from build123d import *

# Parameters (mm, degrees)
F0_W     = 69.85
F0_H     = 120.65
F0_W_2   = 9.525
F0_H_2   = 25.4
F1_DEPTH = 6.35
F3_R     = 11.90625
F4_DEPTH = 12.7
F2_R     = 11.90625
F5_DEPTH = 12.7
F6_W     = 11.43
F6_H     = 88.9
F7_DEPTH = 12.7


with BuildPart() as f1:
    # F0 (on Front) → F1 (new body)
    with BuildSketch(Plane.XZ):
        Rectangle(F0_W, F0_H)
        Rectangle(F0_W_2, F0_H_2, mode=Mode.SUBTRACT)
    extrude(amount=F1_DEPTH)

    # F3 (on Front) → F4 (join)
    with BuildSketch(Plane.XZ):
        with Locations((18.782835, 26.751311)):
            Circle(F3_R)
    extrude(amount=F4_DEPTH)

    # F2 (on Front) → F5 (join)
    with BuildSketch(Plane.XZ):
        with Locations((-17.48186, -7.399299)):
            Circle(F2_R)
    extrude(amount=F5_DEPTH)

    # F6 (on Front) → F7 (join)
    with BuildSketch(Plane.XZ):
        Rectangle(F6_W, F6_H)
    extrude(amount=F7_DEPTH)


solid = f1.part
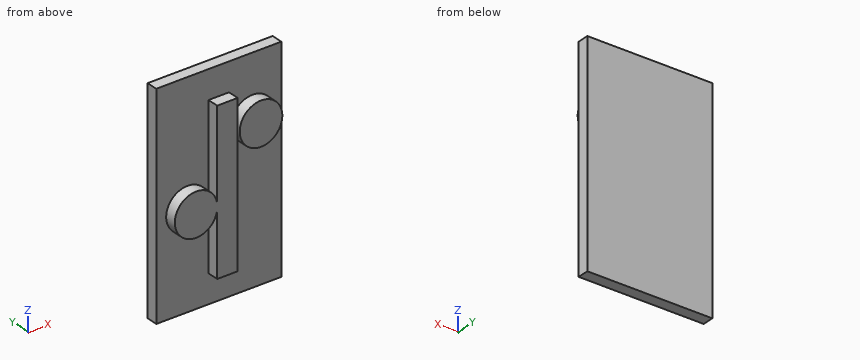
Work out the finished part from the listing and answer in its coordinate system (mm). Coordinates: 2 decimals unless noted, no trailing zeros. Loops run counter-clockwise (first coordinate to the right, second up) from the corner with the lowest first, then second, coordinate; pieces in that order, holes last. Notation, with made-up numbers: M 36.5,63 L 40.5,63 A13 cw 40.5,68 Z; hole C 32,34.25 d7. An arc over 180 degrees is marked long. Answer in a Markdown table with one row per item. Add a question column.
1. Flat-ended cylindrical pins translate along their axes: P1, Ø1, axis at x = 17, y = -8.5, coming from the -Z side; P2, Ø3, axis at x = 1, y = -8.5, coming from the +Z side; P3, Ø5, axis at y = -11, z = -19.5, coming from the -X side; P4, Ø7, axis at y = -9, z = 26.5, coming from the -X side (3 decimals). Find the tip coordinate at first contact, or state that the pin passes through.
2. Find section D-D, the plane z = 36. Write down the section's boundary in (x, y) (3 decimals), then the cut area to 3 significant figures.
3. Find section A-A, the plane z = 7. Write down the section's boundary in (x, y) (3 decimals), then the cut area to 3 significant figures.
4. Find section C-C, the plane x = 1. Write down the section's boundary in (y, z) (3 decimals), then the cut area to 3 significant figures.
5. Consider L1, parallel to Y at x = -24.5, z = 26.5; L2, parallel to X at y = -11.5, z = -27.5 (3 decimals); L3, parallel to X at y = -10.5, z = 33.5 (3 decimals). Determine where each line is inside the solid, lowest interval first.
Reported:
| question | item | result |
|---|---|---|
| 1 | P1 | stops at z = 14.91 |
| 1 | P2 | stops at z = 44.45 |
| 1 | P3 | stops at x = -24.52 |
| 1 | P4 | stops at x = -34.925 |
| 2 | outline | M -34.925,-6.35 L -5.715,-6.35 L -5.715,-12.7 L 5.715,-12.7 L 5.715,-6.35 L 11.285,-6.35 L 11.285,-12.7 L 26.281,-12.7 L 26.281,-6.35 L 34.925,-6.35 L 34.925,0 L -34.925,0 Z |
| 2 | area | 611 mm^2 |
| 3 | outline | M -34.925,-6.35 L -5.715,-6.35 L -5.715,-12.7 L 5.715,-12.7 L 5.715,-6.35 L 34.925,-6.35 L 34.925,0 L -34.925,0 Z |
| 3 | area | 516 mm^2 |
| 4 | outline | M -12.7,-44.45 L -6.35,-44.45 L -6.35,-60.325 L 0,-60.325 L 0,60.325 L -6.35,60.325 L -6.35,44.45 L -12.7,44.45 Z |
| 4 | area | 1,330 mm^2 |
| 5 | L1 | y = -6.35 to 0 |
| 5 | L2 | x = -5.715 to 5.715 |
| 5 | L3 | x = -5.715 to 5.715, 8.974 to 28.592 |
